Check sheet for the modelled part. Datum: model origin and axes. Units: mm. A direction names the side the tool comes from. Round coordinates to 2 decimals unless told otherwise and drop trailing zeros. Order: outer loops, then holes, each group sorted by start corner. A loop starts at its lowest first (then second) coordinate and runs counter-clockwise, first axis right, second up. Notation, with made-up numbers: (53.5, -34) -> (78.5, -34) arc R23 ccw to (78.5, -12) -> close; hole circle Ø10 at (70, 14.5). An arc over 180 degrees is marked (long way). Use CSV: the item, a comma, the result in double quotes.
```python
from build123d import *

# Parameters (mm, degrees)
EXTRUDE_3_DEPTH     = 35
SKETCH_3_R          = 2.1
CUT_EXTRUDE_1_DEPTH = 56.502598264
SKETCH_4_R          = 5
CUT_EXTRUDE_2_DEPTH = 1.7


with BuildPart() as part:
    # 草图1 → 凸台-拉伸3 (new body)
    with BuildSketch(Plane.XY):
        Polygon((0, 0), (34.154700538, 0), (34.154700538, 2), (1.154700538, 2), (-12.845299462, 26.248711306), (-14.577350269, 25.248711306), align=None)
    extrude(amount=EXTRUDE_3_DEPTH)

    # 草图3 → 切除-拉伸1 (cut, through all)
    with BuildSketch(Plane.XZ):
        with Locations((21.5, 27.5)):
            Circle(SKETCH_3_R)
        with Locations((21.5, 7.5)):
            Circle(SKETCH_3_R)
    extrude(amount=-CUT_EXTRUDE_1_DEPTH, mode=Mode.SUBTRACT)

    # 草图4 → 切除-拉伸2 (cut)
    with BuildSketch(Plane(origin=(0, 0, 0), x_dir=(0, 0, 1), z_dir=(-0.8660254037844397, -0.499999999999998, 0))):
        with Locations(Location((27.5, 15, 0), (0, 0, 270))):
            Circle(SKETCH_4_R)
        with Locations(Location((7.5, 15, 0), (0, 0, 270))):
            Circle(SKETCH_4_R)
    extrude(amount=-CUT_EXTRUDE_2_DEPTH, mode=Mode.SUBTRACT)


solid = part.part
```
Q1. Access from +Z, -Z, +X, -X, +Y, -Y to the whole of each face (thin tool, end or side, straight path). Record for faces 1 (the face through (18, 2, 17)), 2 (the face through (6.1, 1.5, 35)).
Result sheet:
face 1,"+Z, -Z, +X, +Y"
face 2,"+Z, +X, -X, +Y, -Y"
Q2. Sectioned sample at A-A, the plane x = 21.5. Enter the section's corners in (y, z).
Result sheet:
outline,"(0, 0) -> (2, 0) -> (2, 5.4) -> (0, 5.4) -> close; (0, 9.6) -> (2, 9.6) -> (2, 25.4) -> (0, 25.4) -> close; (0, 29.6) -> (2, 29.6) -> (2, 35) -> (0, 35) -> close"
Q3. Sectioned sample at C-C, the plane x = 27.5. Enter the section's corners in (y, z).
Result sheet:
outline,"(0, 0) -> (2, 0) -> (2, 35) -> (0, 35) -> close"
Q4. Sectioned sample at D-D, the plane y = 2.75. Enter the section's corners in (x, z), then the cut area to 3 significant figures.
Result sheet:
outline,"(-1.59, 0) -> (0.72, 0) -> (0.72, 35) -> (-1.59, 35) -> close"
area,"80.8 mm^2"
Q5. Sectioned sample at B-B, the plane z = 7.5. Enter the section's corners in (x, y).
Result sheet:
outline,"(-14.58, 25.25) -> (-10, 17.32) -> (-8.53, 18.17) -> (-3.53, 9.51) -> (-5, 8.66) -> (0, 0) -> (19.4, 0) -> (19.4, 2) -> (1.15, 2) -> (-12.85, 26.25) -> close; (23.6, 0) -> (34.15, 0) -> (34.15, 2) -> (23.6, 2) -> close"
Q6. Scan lines: L1, parallel to Z at x = 21.5, y = 1; L2, parallel to Y at x = 18.5, z = 26.5; L3, parallel to Y at x = -4.5, z = 9. Record each from-to range of solid material in increasing order.
Result sheet:
L1,"z = 0 to 5.4, 9.6 to 25.4, 29.6 to 35"
L2,"y = 0 to 2"
L3,"y = 7.79 to 9.21, 11.19 to 11.79"
Q7. Mould release check, pull along Z, two halves, no side actions. Record for faces 3 (the face through (-13.699, 25.756, 17.255)), 4 (the face through (-6.06, 13.9, 7.57)), 5 (the face through (6.1, 1.5, 0)), 6 (the face through (-7.32, 14.35, 22.62)): pulls with the +Z half, pulls with the -Z half, needs draft (parallel to the pull), parting line crosses it, or undercut.
Result sheet:
face 3,"needs draft"
face 4,"undercut"
face 5,"pulls with the -Z half"
face 6,"undercut"
Q8. Go/stop test with flat-tipped pins: pin 1 (12 mm diameter, centred on x = 6, z = 20.5, fed in from +Y); pin 2 (10 mm diameter, centred on x = 17.5, z = 12.5, fed in from +Y); pin 3 (3 mm diameter, centred on y = 19.5, z = 23, fed in from +X); pin 4 (6 mm diameter, centred on x = 7.5, y = 7, fed in from -Z). Record where each tip stops, or that it passes through.
Result sheet:
pin 1,"stops at y = 4"
pin 2,"stops at y = 2"
pin 3,"stops at x = -8.08"
pin 4,"passes through"
